from build123d import *

# Parameters (mm, degrees)
SKETCH_1_W          = 58
SKETCH_1_H          = 25.4
EXTRUDE_1_DEPTH     = 3
SKETCH_2_W          = 8
SKETCH_2_H          = 3
EXTRUDE_2_DEPTH     = 28
SKETCH_3_R          = 3
CUT_EXTRUDE_1_DEPTH = 12
SKETCH_4_R          = 2
CUT_EXTRUDE_2_DEPTH = 22
SKETCH_8_W          = 8
SKETCH_8_H          = 3
CUT_EXTRUDE_3_DEPTH = 28
EXTRUDE_3_DEPTH     = 1
EXTRUDE_4_DEPTH     = 1


with BuildPart() as part:
    # 草图1 → 凸台-拉伸1 (new body)
    with BuildSketch(Plane(origin=(0, 0, 0), x_dir=(1, 0, 0), z_dir=(0, 1, 0))):
        Rectangle(SKETCH_1_W, SKETCH_1_H)
    extrude(amount=EXTRUDE_1_DEPTH)

    # 草图2 → 凸台-拉伸2 (add)
    with BuildSketch(Plane(origin=(0, 3, 0), x_dir=(1, 0, 0), z_dir=(0, 1, 0))):
        with Locations((-24.75, 11.2)):
            Rectangle(SKETCH_2_W, SKETCH_2_H)
        with Locations((24.75, 11.2)):
            Rectangle(SKETCH_2_W, SKETCH_2_H)
        with Locations((-24.75, 0)):
            Rectangle(SKETCH_2_W, SKETCH_2_H)
        with Locations((24.75, 0)):
            Rectangle(SKETCH_2_W, SKETCH_2_H)
    extrude(amount=EXTRUDE_2_DEPTH)

    # 草图3 → 切除-拉伸1 (cut, symmetric)
    with BuildSketch(Plane.XY.offset(-9.7)):
        with Locations((-24.75, 12)):
            Circle(SKETCH_3_R)
        with Locations((-24.75, 22)):
            Circle(SKETCH_3_R)
        with Locations((24.75, 12)):
            Circle(SKETCH_3_R)
        with Locations((24.75, 22)):
            Circle(SKETCH_3_R)
    extrude(amount=CUT_EXTRUDE_1_DEPTH, both=True, mode=Mode.SUBTRACT)

    # 草图4 → 切除-拉伸2 (cut)
    with BuildSketch(Plane(origin=(0, 3, 0), x_dir=(1, 0, 0), z_dir=(0, 1, 0))):
        with Locations((24.75, -7.5)):
            Circle(SKETCH_4_R)
        with Locations((24.75, 7.5)):
            Circle(SKETCH_4_R)
        with Locations((-4.85, 7.5)):
            Circle(SKETCH_4_R)
        with Locations((-4.85, -7.5)):
            Circle(SKETCH_4_R)
    extrude(amount=-CUT_EXTRUDE_2_DEPTH, mode=Mode.SUBTRACT)

    # 草图8 → 切除-拉伸3 (cut)
    with BuildSketch(Plane(origin=(0, 31, 0), x_dir=(1, 0, 0), z_dir=(0, 1, 0))):
        with Locations((-24.75, 11.2)):
            Rectangle(SKETCH_8_W, SKETCH_8_H)
        with Locations((24.75, 11.2)):
            Rectangle(SKETCH_8_W, SKETCH_8_H)
    extrude(amount=-CUT_EXTRUDE_3_DEPTH, mode=Mode.SUBTRACT)

    # 草图9 → 凸台-拉伸3 (add, symmetric)
    with BuildSketch(Plane(origin=(29, 0, 0), x_dir=(0, 0, -1), z_dir=(1, 0, 0))):
        Polygon((-12.7, 3), (-1.5, 3), (-1.5, 31), (1.5, 31), (1.5, 3), (12.7, 3), (12.7, 0), (-12.7, 0), align=None)
    extrude(amount=EXTRUDE_3_DEPTH, both=True)

    # 草图10 → 凸台-拉伸4 (add, symmetric)
    with BuildSketch(Plane.ZY.offset(29)):
        Polygon((-12.7, 3), (-1.5, 3), (-1.5, 31), (1.5, 31), (1.5, 3), (12.7, 3), (12.7, 0), (-12.7, 0), align=None)
    extrude(amount=EXTRUDE_4_DEPTH, both=True)


solid = part.part
For this review, take the finished solid that the model builds, in its own axes (mm). A direction names the side the tool comes from. Round coordinates to 2 decimals unless told otherwise and drop trailing zeros. Order: outer loops, then holes, each group sorted by start corner. A loop starts at its lowest first (then second) coordinate and runs counter-clockwise, first axis right, second up. Notation, with made-up numbers: M 82,28.5 L 125,28.5 A21 ccw 125,35.5 Z; hole C -18,82.25 d1. An arc over 180 degrees is marked long. Use a Markdown table: item, result. Add a question column.
Item 1: Add section D-D, the plane x = 24.75. Give the boundary of the cut face in (y, z), then the cut area to 3 significant figures.
Item 2: Add section C-C, the plane y = 22. Give the boundary of the cut face in (x, z), then the cut area to 3 significant figures.
Item 3: Mouldability with a two-part tool opening along Y and no side actions: class faces 1 (the flat face through (0, 1, -12.7)), 2 (the cylindrical face through (-27.747, 12.132, -0.021)), 3 (the cylindrical face through (21.753, 12.132, -0.021)), 4 (the flat face through (0, 0, 0)) as released by +Y, released by -Y, zero draft, split by the parting line, or undercut.
Item 4: Add section B-B, the plane z = 7.5. Give the boundary of the cut face in (x, y).
Item 5: To check wall thickness, follow line 1 along X through (y, z) = (12, 0.65); line 2 along X through (y, z) = (0.9, 7.5); line 3 along Y through (x, z) = (24.75, 0.9). State the ranges of each line that lie inside material, in increasing order.
Item 6: Tool access review of faces 5 (the flat face through (25, 17, -1.5)), 6 (the flat face through (25, 17, 1.5)), 7 (the flat face through (20.75, 17, 0)): name each direction out of +Z, -Z, +X, -X, +Y, -Y from which nothing blocks a thin tool from reaching the whole face with its end or side.
Item 7: Add section A-A, the plane x = -4.85. Give the boundary of the cut face in (y, z).
Item 8: Insertion check: pin 1 (5 mm diameter, centred on x = -4.85, z = 7.5, fed in from +Y); pin 2 (4 mm diameter, centred on x = 19, y = 20, fed in from +Z); pin 3 (10 mm diameter, centred on x = -26, y = 12.5, fed in from -Z). Each pin has a flat end and moves straight along its axis. Give the tip position at first contact, or say it passes through.
Geometry results:
| question | item | result |
|---|---|---|
| 1 | outline | M 0,-12.7 L 3,-12.7 L 3,-9.5 L 0,-9.5 Z; M 0,-5.5 L 3,-5.5 L 3,-1.5 L 9,-1.5 L 9,1.5 L 3,1.5 L 3,5.5 L 0,5.5 Z; M 0,9.5 L 3,9.5 L 3,12.7 L 0,12.7 Z; M 15,-1.5 L 19,-1.5 L 19,1.5 L 15,1.5 Z; M 25,-1.5 L 31,-1.5 L 31,1.5 L 25,1.5 Z |
| 1 | area | 100 mm² |
| 2 | outline | M -30,-1.5 L -27.75,-1.5 L -27.75,1.5 L -30,1.5 Z; M -21.75,-1.5 L -20.75,-1.5 L -20.75,1.5 L -21.75,1.5 Z; M 20.75,-1.5 L 21.75,-1.5 L 21.75,1.5 L 20.75,1.5 Z; M 27.75,-1.5 L 30,-1.5 L 30,1.5 L 27.75,1.5 Z |
| 2 | area | 19.5 mm² |
| 3 | face 1 | zero draft |
| 3 | face 2 | undercut |
| 3 | face 3 | undercut |
| 3 | face 4 | released by -Y |
| 4 | outline | M -30,0 L -6.85,0 L -6.85,3 L -30,3 Z; M -2.85,0 L 22.75,0 L 22.75,3 L -2.85,3 Z; M 26.75,0 L 30,0 L 30,3 L 26.75,3 Z |
| 5 | line 1 | x = -30 to -27.75, -21.75 to -20.75, 20.75 to 21.75, 27.75 to 30 |
| 5 | line 2 | x = -30 to -6.85, -2.85 to 22.75, 26.75 to 30 |
| 5 | line 3 | y = 0 to 9, 15 to 19, 25 to 31 |
| 6 | face 5 | -Z, +X, -X, +Y |
| 6 | face 6 | +Z, +X, -X, +Y |
| 6 | face 7 | +Z, -Z, +Y |
| 7 | outline | M 0,-12.7 L 3,-12.7 L 3,-9.5 L 0,-9.5 Z; M 0,-5.5 L 3,-5.5 L 3,5.5 L 0,5.5 Z; M 0,9.5 L 3,9.5 L 3,12.7 L 0,12.7 Z |
| 8 | pin 1 | stops at y = 3 |
| 8 | pin 2 | stops at z = 1.5 |
| 8 | pin 3 | stops at z = -1.5 |
